Check sheet for the modelled part. Datum: model origin and axes. Units: mm. A direction names the side the tool comes from. Give positions to 0.01 mm unless a question says otherwise; leave off trailing zeros. Order: outer loops, then holes, each group sorted by start corner. A loop starts at its lowest first (then second) coordinate and runs counter-clockwise, first axis right, second up. Notation, with made-up numbers: M -39,4 L 15,4 A26 cw 15,33 Z; hole C 43,13.25 d5. An arc over 180 degrees is marked long. Return JSON: item names as keys, results as strings. Group by question number.
from build123d import *

# Parameters (mm, degrees)
F1_DEPTH = 50
F2_R     = 3
F3_R     = 25
F4_DEPTH = 30


with BuildPart() as f1:
    # F0 (on Front) → F1 (new body)
    with BuildSketch(Plane.XZ):
        with BuildLine():
            Line((54.576429, 67.460465), (-20.423571, 67.460465))
            ThreePointArc((-20.423571, 67.460465), (-38.101241, 60.138135), (-45.423571, 42.460465))
            Line((-45.423571, 42.460465), (-45.423571, -32.539535))
            Line((-45.423571, -32.539535), (29.576429, -32.539535))
            ThreePointArc((29.576429, -32.539535), (47.254099, -25.217204), (54.576429, -7.539535))
            Line((54.576429, -7.539535), (54.576429, 67.460465))
        make_face()
    extrude(amount=F1_DEPTH)

    # F2
    f2_edges = [f1.edges().sort_by_distance(p)[0] for p in [
        (17.076429, -50, 67.460465),
        (-38.101241, -50, 60.138135),
        (-45.423571, -50, 4.960465),
        (-7.923571, -50, -32.539535),
        (47.254099, -50, -25.217204),
        (54.576429, -50, 29.960465),
    ]]
    fillet(f2_edges, radius=F2_R)

    # F3 (on face) → F4 (cut)
    with BuildSketch(Plane.XZ.offset(50)):
        with Locations((6.760165, 18.145708)):
            Circle(F3_R)
    extrude(amount=-F4_DEPTH, mode=Mode.SUBTRACT)


solid = f1.part
1) Sectioned sample at C-C on z = 16.5. Record the boundary of the cut face in (x, y), then the cut area to 3 significant figures.
2) Material ranges on line 1 along X through (y, z) = (-29.5, 10.5); line 2 along Y through (x, z) = (16.5, 28.5); line 3 along X through (y, z) = (-26.5, 10), recorded low to high.
3) Tool access check on faces 1 (the face through (-17, -50, 8)), 2 (the face through (6, -20, 18)). Record the directions out of +Z, -Z, +X, -X, +Y, -Y that give a thin tool (end or side, any length) a straight path to the whole face; none if there is none.
4) Depth check by flat-ended pin: P1, Ø1.5, axis at y = -11, z = -12, coming from the +X side; P2, Ø1, axis at x = -32, z = 45.5, coming from the +Y side; P3, Ø4, axis at x = -28, y = -27.5, coming from the +Z side. Enter the tip coordinate at first touch or a pass-through.
5) Sectioned sample at D-D on y = -40. Record the boundary of the cut face in (x, z).
6) Sectioned sample at A-A on x = -3. Record the boundary of the cut face in (y, z).
7) Sectioned sample at B-B on y = -8. Record the boundary of the cut face in (x, z).
Reply:
{
 "1": {"outline": "M -45.42,-47 A3 ccw -42.42,-50 L -18.19,-50 L -18.19,-20 L 31.71,-20 L 31.71,-50 L 51.58,-50 A3 ccw 54.58,-47 L 54.58,0 L -45.42,0 Z", "area": "3,500 mm^2"},
 "2": {"line 1": "-45.42 to -17.04, 30.56 to 54.58", "line 2": "-20 to 0", "line 3": "-45.42 to -16.88, 30.4 to 54.58"},
 "3": {"face 1": "+Z, -Z, +X, -X, -Y", "face 2": "-Y"},
 "4": {"P1": "x = 54.3", "P2": "y = 0", "P3": "z = 66.83"},
 "5": {"outline": "M -45.42,-32.54 L 29.58,-32.54 A25 ccw 54.58,-7.54 L 54.58,67.46 L -20.42,67.46 A25 ccw -45.42,42.46 Z; hole C 6.76,18.15 d50"},
 "6": {"outline": "M -50,-29.54 A3 ccw -47,-32.54 L 0,-32.54 L 0,67.46 L -47,67.46 A3 ccw -50,64.46 L -50,41.16 L -20,41.16 L -20,-4.87 L -50,-4.87 Z"},
 "7": {"outline": "M -45.42,-32.54 L 29.58,-32.54 A25 ccw 54.58,-7.54 L 54.58,67.46 L -20.42,67.46 A25 ccw -45.42,42.46 Z"}
}
